Geometry: see drawing. Coordinates: mm, zero at the bounding-box minimum. A direction names the side the tool comes from. Round coordinates to 2 decimals unless told otherwise and drop trailing zeros. Loops run counter-clockwise (first coordinate to the right, second up) from the corner with the lowest first, then second, coordinate; pieces in that order, holes last. Notation, with made-up numbers: (-37.5, 57) - (-4.5, 57) arc R9 cw to (-4.5, 66) - close; hole circle Ø5 at (8.5, 64). An arc over 180 degrees is marked (long way). Write item = value, one per line. Start each with the question number.
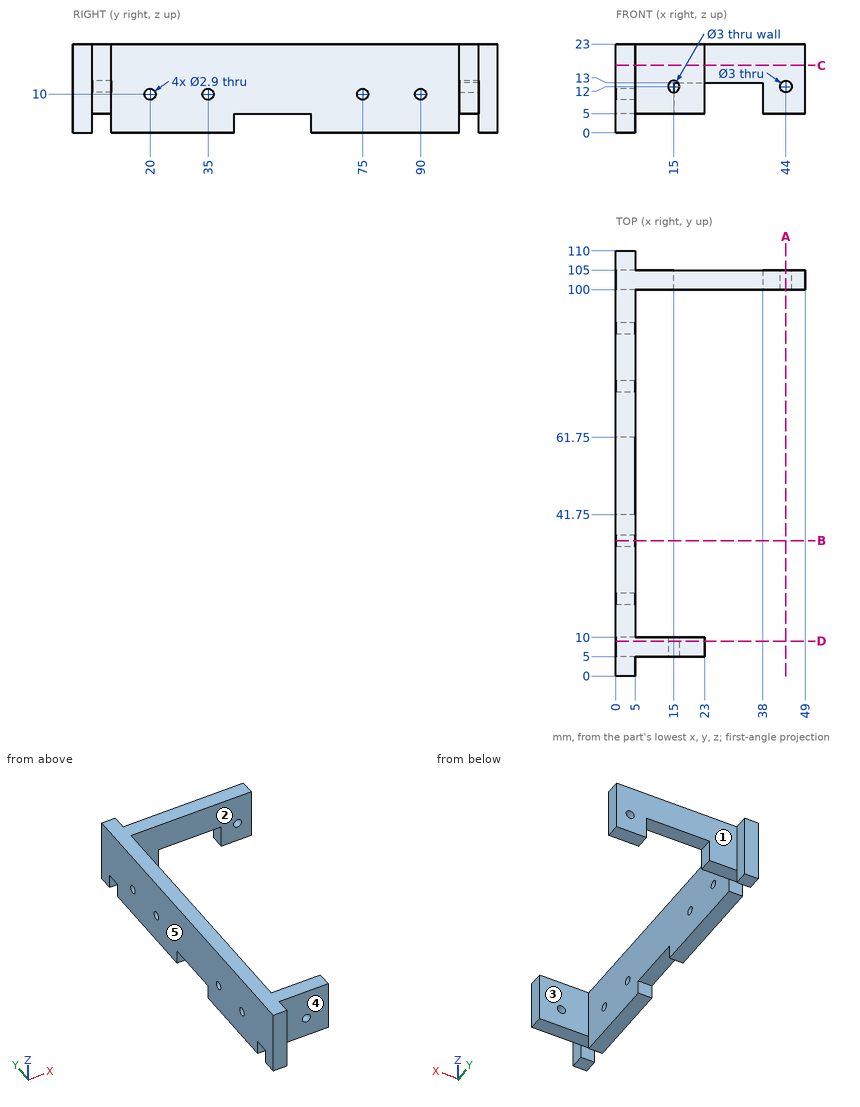
(1) Mould query, pull axis Y, two halves, no side actions, for the marked faces 3, 4 and 5. Classes: +Y half, -Y half, draft (parallel to the pull), parting line (faces both ways), or undercut.
(2) Cut plane D-D (y = 9). Output: boundary loops of the cut face in (x, z).
(3) Access query for the marked faces 1 and 2. Directions: +Z, -Z, +X, -X, +Y, -Y. A direction counts if a zero-diameter tool reaches every point of the face in a straight line with its end or side. Return the directions, or none.
(4) Material intervals for line 1 along X through (y, z) = (103.7, 12); line 2 along Z through (x, y) = (2.85, 20); line 3 along Y through (x, z) = (20, 20), sorted ascending. Write a range as from..to.
(5) Cut plane B-B (y = 35). Output: boundary loops of the cut face in (x, z), and give its area (4 significant figures).
(6) Cut plane C-C (z = 17.5). Output: boundary loops of the cut face in (x, y).
(7) Pin query (flat end, axial travel): P1, Ø5.5, axis at x = 16.5, z = 10.5, coming from the -Y side; P2, Ø4, axis at x = 2.5, z = 2, coming from the -Y side; P3, Ø4, axis at y = 90, z = 10, coming from the +X side; P4, Ø2.5, axis at y = 35, z = 10, coming from the -X side. Return the tip coordinate at first contact, or that it passes through.
(8) Cut plane A-A (x = 44). Output: boundary loops of the cut face in (y, z), and give its area (3 significant figures).
Solution:
q1.face_3 = undercut
q1.face_4 = -Y half
q1.face_5 = draft
q2.outline = (0, 5) - (23, 5) - (23, 23) - (0, 23) - close; hole circle Ø3 at (15, 12)
q3.face_1 = +Z, -Z, +X, +Y
q3.face_2 = +Z, -Z, +X
q4.line_1 = 0..15, 38..42.5, 45.5..49
q4.line_2 = 0..8.55, 11.45..23
q4.line_3 = 5..10, 100..105
q5.outline = (0, 0) - (5, 0) - (5, 8.55) - (0, 8.55) - close; (0, 11.45) - (5, 11.45) - (5, 23) - (0, 23) - close
q5.area = 100.5 mm^2
q6.outline = (0, 0) - (5, 0) - (5, 5) - (23, 5) - (23, 10) - (5, 10) - (5, 100) - (49, 100) - (49, 105) - (5, 105) - (5, 110) - (0, 110) - close
q7.P1 = 5
q7.P2 = 0
q7.P3 = 5
q7.P4 = through
q8.outline = (100, 5) - (105, 5) - (105, 10.5) - (100, 10.5) - close; (100, 13.5) - (105, 13.5) - (105, 23) - (100, 23) - close
q8.area = 75.0 mm^2
